```python
from build123d import *

# Parameters (mm, degrees)
SKETCH_1_R             = 63.5
EXTRUDE_1_DEPTH        = 50
FILLET_1_R             = 10
SKETCH_2_R             = 5
EXTRUDE_2_DEPTH        = 20
EXTRUDE_START          = 20
SKETCH_3_R             = 5
EXTRUDE_3_DEPTH        = 20
EXTRUDE_START_2        = 3
SKETCH_4_R             = 5
EXTRUDE_4_DEPTH        = 3
PATTERN_LINEAR_1_COUNT = 2
PATTERN_LINEAR_1_PITCH = 63
SKETCH_5_W             = 52.384505053
SKETCH_5_H             = 66
EXTRUDE_5_DEPTH        = 3
SKETCH_6_R             = 5
CUT_EXTRUDE_1_DEPTH    = 3
SKETCH_7_W             = 108.179639097
SKETCH_7_H             = 94.795773282
SKETCH_7_R             = 5
EXTRUDE_6_DEPTH        = 3


with BuildPart() as part:
    # 草图1 → 凸台-拉伸1 (new body)
    with BuildSketch(Plane.XY):
        Circle(SKETCH_1_R)
    extrude(amount=EXTRUDE_1_DEPTH)

    # 圆角1
    fillet_1_edges = [part.edges().sort_by_distance(p)[0] for p in [
        (-63.5, 0, 0),
        (-63.5, 0, 50),
    ]]
    fillet(fillet_1_edges, radius=FILLET_1_R)

    # 草图2 → 凸台-拉伸2 (add)
    with BuildSketch(Plane(origin=(0, 0, 0), x_dir=(-1, 0, 0), z_dir=(0, 0, -1))):
        with Locations(Location((0, 0, 0), (0, 0, 180))):
            Circle(SKETCH_2_R)
    extrude(amount=EXTRUDE_2_DEPTH)

    # 草图3 → 凸台-拉伸3 (add)
    with BuildSketch(Plane.XY.offset(50).offset(EXTRUDE_START)):
        Circle(SKETCH_3_R)
    extrude(amount=-EXTRUDE_3_DEPTH)

    # 草图4 → 凸台-拉伸4 (add)
    with BuildSketch(Plane.XY.offset(55).offset(EXTRUDE_START_2)):
        Polygon((-14.847710206, -30.641134437), (19.008851919, -30.641134437), (19.008851919, 76.850518215), (-33.375653134, 76.850518215), (-14.847710206, -29.89657058), align=None)
        Circle(SKETCH_4_R, mode=Mode.SUBTRACT)
    extrude_4 = extrude(amount=-EXTRUDE_4_DEPTH)

    # 阵列(线性)1: 凸台-拉伸4 ×2
    with Locations(*[(0, 0, -i * PATTERN_LINEAR_1_PITCH) for i in range(1, PATTERN_LINEAR_1_COUNT)]):
        add(extrude_4)

    # 草图5 → 凸台-拉伸5 (add)
    with BuildSketch(Plane(origin=(0, 76.850518215, 0), x_dir=(1, 0, 0), z_dir=(0, 1, 0))):
        with Locations((-7.183400608, -25)):
            Rectangle(SKETCH_5_W, SKETCH_5_H)
    extrude(amount=EXTRUDE_5_DEPTH)

    # 草图6 → 切除-拉伸1 (cut)
    with BuildSketch(Plane(origin=(0, 79.850518215, 0), x_dir=(1, 0, 0), z_dir=(0, 1, 0))):
        with Locations(Location((-7.183400607, -25, 0), (0, 0, 270))):
            Circle(SKETCH_6_R)
    extrude(amount=-CUT_EXTRUDE_1_DEPTH, mode=Mode.SUBTRACT)

    # 草图7 → 凸台-拉伸6 (add)
    with BuildSketch(Plane(origin=(0, 79.850518215, 0), x_dir=(1, 0, 0), z_dir=(0, 1, 0)).offset(EXTRUDE_START_2)):
        with Locations((-7.183400607, -25)):
            Rectangle(SKETCH_7_W, SKETCH_7_H)
        with Locations(Location((-53.277526454, 15.391411359, 0), (0, 0, 270))):
            Circle(SKETCH_7_R, mode=Mode.SUBTRACT)
        with Locations(Location((-53.277526454, -65.391411359, 0), (0, 0, 270))):
            Circle(SKETCH_7_R, mode=Mode.SUBTRACT)
        with Locations(Location((38.910725239, -65.391411359, 0), (0, 0, 270))):
            Circle(SKETCH_7_R, mode=Mode.SUBTRACT)
        with Locations(Location((38.910725239, 15.391411359, 0), (0, 0, 270))):
            Circle(SKETCH_7_R, mode=Mode.SUBTRACT)
        with Locations(Location((-7.183400607, -25, 0), (0, 0, 270))):
            Circle(SKETCH_7_R, mode=Mode.SUBTRACT)
    extrude(amount=-EXTRUDE_6_DEPTH)


solid = part.part
```
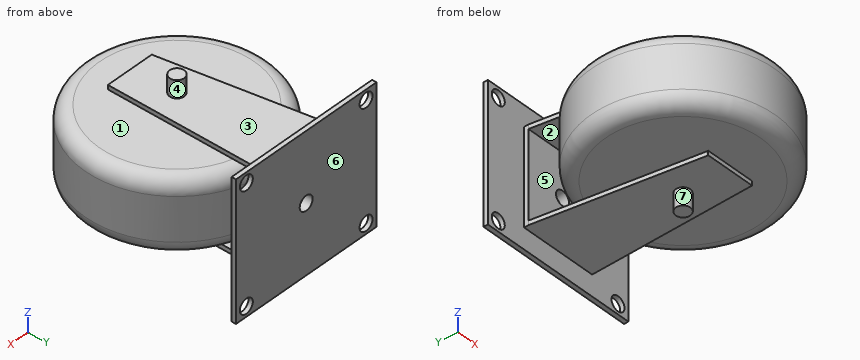
Here's how the part is built. I have some questions about the finished solid (model axes, mm). Face numbers are marked on the shaded views. A direction names the side the tool comes from. Coordinates: 2 decimals unless noted, no trailing zeros. Order: outer loops, then holes, each group sorted by start corner. A loop starts at its lowest first (then second) coordinate and runs counter-clockwise, first axis right, second up. Notation, with made-up numbers: (69.5, -28) - (99.5, -28) arc R24 cw to (99.5, 4) - close; hole circle Ø7 at (81.25, 80). An arc over 180 degrees is marked (long way). One line per question, with ' | ' between items. Start each with the question number.
1. If we section it at A-A (z = 25): Write out the boundary of the cut face in (x, y).
2. If we mould it in two halves opening along Z, with no side actions, what happens to the marked faces 1, 2, 3 and 4? For each: released by +Z, released by -Z, zero draft, split by the parting line, or undercut.
3. Please list where these lines run through material, in increasing order: line 1 along Z through (x, y) = (5.5, -4); line 2 along X through (y, z) = (79.8, 25); line 3 along X through (y, z) = (81.5, 25). Write a range as [from, to].
4. I'm going to push flat-ended pins straight in: pin 1 Ø1 at (y, z) = (54.5, 29) entering from +X; pin 2 Ø5 at (x, y) = (12, -32.5) entering from -Z; pin 3 Ø1 at (y, z) = (-26, 7) entering from +X; pin 4 Ø11.5 at (x, z) = (-53.28, -15.39) entering from +Y. Where does each tip first touch, or does it pass through?
5. If we section it at B-B (z = 8): Write out the boundary of the cut face in (x, y), and give its area (3 significant figures).
6. Which directions (+Z, -Z, +X, -X, +Y, -Y) give clear straight access to the entire face, cutting with the end or side of a thin tool? Please do the marked faces 5, 6 and 7.
7. If we section it at D-D (x = 41.5): Give the number of separate pieces and of enclosed holes in the cut face, and give its area (3 significant figures).
Model answer:
1) outline: circle Ø127 at (0, 0); (-61.27, 79.85) - (-33.38, 79.85) - (-33.38, 76.85) - (-12.18, 76.85) - (-12.18, 82.85) - (-61.27, 82.85) - close; (-2.18, 76.85) - (19.01, 76.85) - (19.01, 79.85) - (46.91, 79.85) - (46.91, 82.85) - (-2.18, 82.85) - close
2) face 1: undercut | face 2: undercut | face 3: released by +Z | face 4: zero draft
3) line 1: z = [-8, -5], [0, 50], [55, 58] | line 2: x = [-33.38, -12.18], [-2.18, 19.01] | line 3: x = [-61.27, -12.18], [-2.18, 46.91]
4) pin 1: stops at x = 33.41 | pin 2: stops at z = -8 | pin 3: stops at x = 57.71 | pin 4: stops at y = 82.85
5) outline: circle Ø126.6 at (0, 0); (-61.27, 79.85) - (-33.38, 79.85) - (-33.38, 76.85) - (19.01, 76.85) - (19.01, 79.85) - (46.91, 79.85) - (46.91, 82.85) - (-61.27, 82.85) - close | area: 13,100 mm²
6) face 5: +X, -X | face 6: +Z, -Z, +X, -X, +Y | face 7: -Z
7) separate pieces: 4 | enclosed holes: 0 | area: 4,920 mm²
